Geometry check sheet. Reference: the model listing, model coordinates, mm. Give positions to 0.01 mm unless a question says otherwise; leave off trailing zeros. Order: outer loops, then holes, each group sorted by start corner. A loop starts at its lowest first (then second) coordinate and runs counter-clockwise, first axis right, second up. Notation, with made-up numbers: M -28.75,64 L 2.25,64 A23 ccw 2.25,88 Z; hole C 87,11 d10. An arc over 180 degrees is marked long. Answer as CSV lines item,"result".
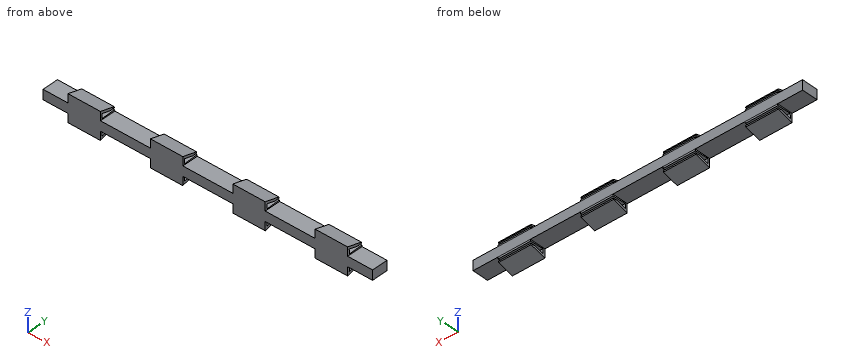
from build123d import *

# Parameters (mm, degrees)
CLIP_1_DEPTH           = 10
CENTER_BEAM_DEPTH      = 177.8
CENTER_BEAM_DEPTH_BACK = 25.4
SKETCH4_W              = 6.003992509
SKETCH4_H              = 9.824299843
LPATTERN1_START        = 40.8
LPATTERN1_DEPTH        = 20
LPATTERN1_START_2      = 91.6
LPATTERN1_2_DEPTH      = 20
LPATTERN1_START_3      = 142.4
LPATTERN1_3_DEPTH      = 20


# Read off the part's stored shape, not the designer's step: LPattern1
with BuildPart() as part:
    # Sketch1 → Clip _1 (new, symmetric)
    with BuildSketch(Plane(origin=(0, 0, 0), x_dir=(0, 0, -1), z_dir=(1, 0, 0))):
        with BuildLine():
            Line((6.081551938, 6.841542851), (7.61911384, 1.103283712))
            Line((7.61911384, 1.103283712), (4.687365208, 1.256930148))
            Line((4.687365208, 1.256930148), (5.127959845, 9.663976652))
            Line((5.127959845, 9.663976652), (4.1299561, 9.824299843))
            Line((4.1299561, 9.824299843), (-1.874036409, 9.824299843))
            Line((-1.874036409, 9.824299843), (-2.872040155, 9.663976652))
            Line((-2.872040155, 9.663976652), (-2.431445517, 1.256930148))
            Line((-2.431445517, 1.256930148), (-5.36319415, 1.103283712))
            Line((-5.36319415, 1.103283712), (-3.825632248, 6.841542851))
            Line((-3.825632248, 6.841542851), (-3.879292118, 7.86543416))
            ThreePointArc((-3.879292118, 7.86543416), (-4.194581765, 8.149322234), (-3.910693691, 8.464611881))
            Line((-3.910693691, 8.464611881), (-3.964353561, 9.488503191))
            Line((-3.964353561, 9.488503191), (-4.701004321, 9.370164756))
            Line((-4.701004321, 9.370164756), (-7.2117324, 0))
            Line((-7.2117324, 0), (-2.365572599, 0))
            Line((-2.365572599, 0), (4.62149229, 0))
            Line((4.62149229, 0), (9.46765209, 0))
            Line((9.46765209, 0), (6.956924011, 9.370164756))
            Line((6.956924011, 9.370164756), (6.220273251, 9.488503191))
            Line((6.220273251, 9.488503191), (6.166613382, 8.464611881))
            ThreePointArc((6.166613382, 8.464611881), (6.450501455, 8.149322234), (6.135211808, 7.86543416))
            Line((6.135211808, 7.86543416), (6.081551938, 6.841542851))
        make_face()
    extrude(amount=CLIP_1_DEPTH, both=True)

    # Sketch4 → Center beam (add, two sides: drawn at the far end of the back side and taken through both)
    with BuildSketch(Plane(origin=(0, 0, 0), x_dir=(0, 0, -1), z_dir=(1, 0, 0)).offset(-CENTER_BEAM_DEPTH_BACK)):
        with Locations((1.127959845, 4.912149922)):
            Rectangle(SKETCH4_W, SKETCH4_H)
    extrude(amount=CENTER_BEAM_DEPTH + CENTER_BEAM_DEPTH_BACK)

    # LPattern1 outline → LPattern1 (add)
    with BuildSketch(Plane.YZ.offset(LPATTERN1_START)):
        with BuildLine():
            Line((0, -4.1299561), (0, -9.46765209))
            Line((0, -9.46765209), (9.370164756, -6.956924011))
            Line((9.370164756, -6.956924011), (9.488503191, -6.220273251))
            Line((9.488503191, -6.220273251), (8.464611881, -6.166613382))
            ThreePointArc((8.464611881, -6.166613382), (8.149322234, -6.450501455), (7.86543416, -6.135211808))
            Line((7.86543416, -6.135211808), (6.841542851, -6.081551938))
            Line((6.841542851, -6.081551938), (1.103283712, -7.61911384))
            Line((1.103283712, -7.61911384), (1.256930148, -4.687365208))
            Line((1.256930148, -4.687365208), (9.663976652, -5.127959845))
            Line((9.663976652, -5.127959845), (9.824299843, -4.1299561))
            Line((9.824299843, -4.1299561), (0, -4.1299561))
        make_face()
        with BuildLine():
            Line((0, 7.2117324), (0, 1.874036409))
            Line((0, 1.874036409), (9.824299843, 1.874036409))
            Line((9.824299843, 1.874036409), (9.663976652, 2.872040155))
            Line((9.663976652, 2.872040155), (1.256930148, 2.431445517))
            Line((1.256930148, 2.431445517), (1.103283712, 5.36319415))
            Line((1.103283712, 5.36319415), (6.841542851, 3.825632248))
            Line((6.841542851, 3.825632248), (7.86543416, 3.879292118))
            ThreePointArc((7.86543416, 3.879292118), (8.149322234, 4.194581765), (8.464611881, 3.910693691))
            Line((8.464611881, 3.910693691), (9.488503191, 3.964353561))
            Line((9.488503191, 3.964353561), (9.370164756, 4.701004321))
            Line((9.370164756, 4.701004321), (0, 7.2117324))
        make_face()
    extrude(amount=LPATTERN1_DEPTH)

    # LPattern1 2 outline → LPattern1 2 (add)
    with BuildSketch(Plane.YZ.offset(LPATTERN1_START_2)):
        with BuildLine():
            Line((0, -4.1299561), (0, -9.46765209))
            Line((0, -9.46765209), (9.370164756, -6.956924011))
            Line((9.370164756, -6.956924011), (9.488503191, -6.220273251))
            Line((9.488503191, -6.220273251), (8.464611881, -6.166613382))
            ThreePointArc((8.464611881, -6.166613382), (8.149322234, -6.450501455), (7.86543416, -6.135211808))
            Line((7.86543416, -6.135211808), (6.841542851, -6.081551938))
            Line((6.841542851, -6.081551938), (1.103283712, -7.61911384))
            Line((1.103283712, -7.61911384), (1.256930148, -4.687365208))
            Line((1.256930148, -4.687365208), (9.663976652, -5.127959845))
            Line((9.663976652, -5.127959845), (9.824299843, -4.1299561))
            Line((9.824299843, -4.1299561), (0, -4.1299561))
        make_face()
        with BuildLine():
            Line((0, 7.2117324), (0, 1.874036409))
            Line((0, 1.874036409), (9.824299843, 1.874036409))
            Line((9.824299843, 1.874036409), (9.663976652, 2.872040155))
            Line((9.663976652, 2.872040155), (1.256930148, 2.431445517))
            Line((1.256930148, 2.431445517), (1.103283712, 5.36319415))
            Line((1.103283712, 5.36319415), (6.841542851, 3.825632248))
            Line((6.841542851, 3.825632248), (7.86543416, 3.879292118))
            ThreePointArc((7.86543416, 3.879292118), (8.149322234, 4.194581765), (8.464611881, 3.910693691))
            Line((8.464611881, 3.910693691), (9.488503191, 3.964353561))
            Line((9.488503191, 3.964353561), (9.370164756, 4.701004321))
            Line((9.370164756, 4.701004321), (0, 7.2117324))
        make_face()
    extrude(amount=LPATTERN1_2_DEPTH)

    # LPattern1 3 outline → LPattern1 3 (add)
    with BuildSketch(Plane.YZ.offset(LPATTERN1_START_3)):
        with BuildLine():
            Line((0, -4.1299561), (0, -9.46765209))
            Line((0, -9.46765209), (9.370164756, -6.956924011))
            Line((9.370164756, -6.956924011), (9.488503191, -6.220273251))
            Line((9.488503191, -6.220273251), (8.464611881, -6.166613382))
            ThreePointArc((8.464611881, -6.166613382), (8.149322234, -6.450501455), (7.86543416, -6.135211808))
            Line((7.86543416, -6.135211808), (6.841542851, -6.081551938))
            Line((6.841542851, -6.081551938), (1.103283712, -7.61911384))
            Line((1.103283712, -7.61911384), (1.256930148, -4.687365208))
            Line((1.256930148, -4.687365208), (9.663976652, -5.127959845))
            Line((9.663976652, -5.127959845), (9.824299843, -4.1299561))
            Line((9.824299843, -4.1299561), (0, -4.1299561))
        make_face()
        with BuildLine():
            Line((0, 7.2117324), (0, 1.874036409))
            Line((0, 1.874036409), (9.824299843, 1.874036409))
            Line((9.824299843, 1.874036409), (9.663976652, 2.872040155))
            Line((9.663976652, 2.872040155), (1.256930148, 2.431445517))
            Line((1.256930148, 2.431445517), (1.103283712, 5.36319415))
            Line((1.103283712, 5.36319415), (6.841542851, 3.825632248))
            Line((6.841542851, 3.825632248), (7.86543416, 3.879292118))
            ThreePointArc((7.86543416, 3.879292118), (8.149322234, 4.194581765), (8.464611881, 3.910693691))
            Line((8.464611881, 3.910693691), (9.488503191, 3.964353561))
            Line((9.488503191, 3.964353561), (9.370164756, 4.701004321))
            Line((9.370164756, 4.701004321), (0, 7.2117324))
        make_face()
    extrude(amount=LPATTERN1_3_DEPTH)


solid = part.part
(1) Material ranges on line 1 (X direction, y = 8.25, z = 4.25); line 2 (Z direction, x = 110.5, y = 5) (3 decimals); line 3 (Z direction, x = 60, y = 7.25), recorded low to high.
The answers:
line 1,"x = -10 to 10, 40.8 to 60.8, 91.6 to 111.6, 142.4 to 162.4"
line 2,"z = -8.128 to -6.575, -4.884 to 2.628, 4.319 to 5.872"
line 3,"z = -7.53 to -6.1, -5 to 2.75, 3.85 to 5.27"
(2) Section check A-A on x = 156. Enter the section's corners in (y, z) (1 decimal).
The answers:
outline,"M 0,-9.5 L 9.4,-7 L 9.5,-6.2 L 8.5,-6.2 A0.3 cw 7.9,-6.1 L 6.8,-6.1 L 1.1,-7.6 L 1.3,-4.7 L 9.7,-5.1 L 9.8,-4.1 L 9.8,1.9 L 9.7,2.9 L 1.3,2.4 L 1.1,5.4 L 6.8,3.8 L 7.9,3.9 A0.3 cw 8.5,3.9 L 9.5,4 L 9.4,4.7 L 0,7.2 Z"
(3) Section check B-B on y = 3.75. State how many separate pieces and enclosed holes the cut face has, then the cut area to 3 significant figures.
The answers:
separate pieces,"9"
enclosed holes,"0"
area,"1,580 mm2"
(4) Section check C-C on x = 73. Enter the section's corners in (y, z), then the cut area to 3 significant figures.
The answers:
outline,"M 0,-4.13 L 9.82,-4.13 L 9.82,1.87 L 0,1.87 Z"
area,"59.0 mm2"
(5) Gauge pin test, flat ends, axial feed: P1, Ø4.5, axis at y = 6, z = 5, coming from the -X side; P2, Ø1.6, axis at y = 4, z = -7.5, coming from the +X side; P3, Ø3, axis at x = 32.5, y = 3, coming from the +Z side. Record the tip position at first contact, or that the pin passes through.
The answers:
P1,"stops at x = -10"
P2,"stops at x = 162.4"
P3,"stops at z = 1.87"
